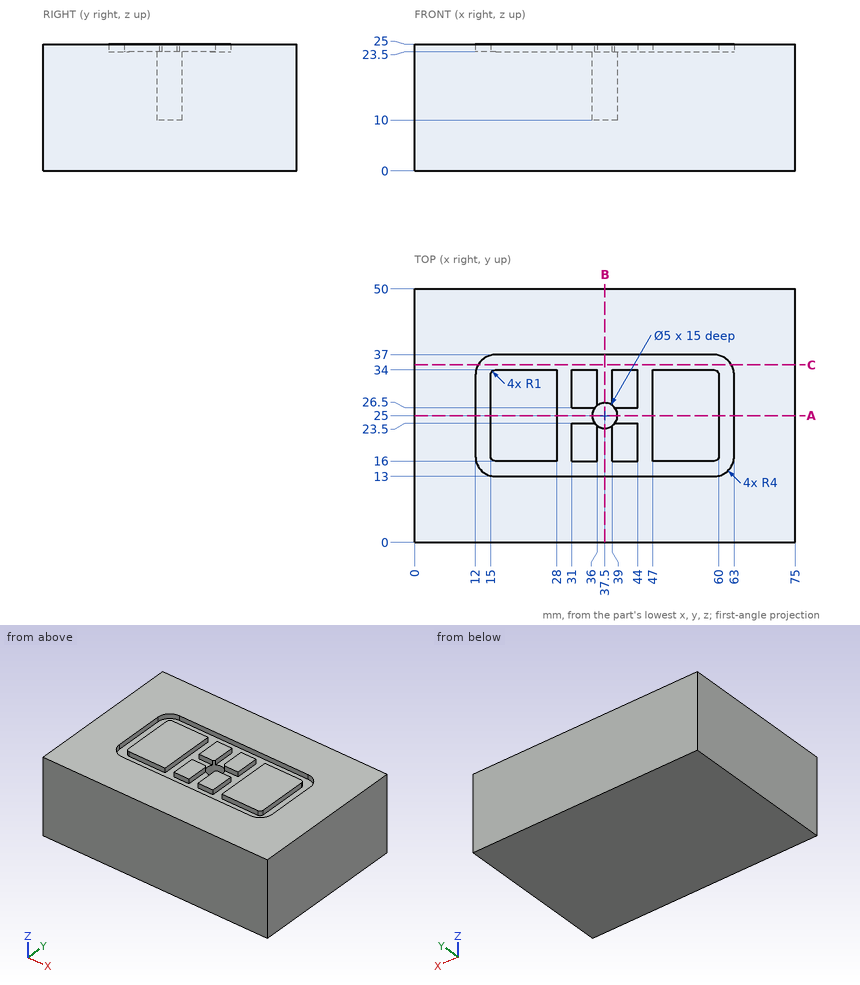
Input: dimensioned drawing with shaded views. Units: mm. Origin: part minimum x, y, z. Coordinates: 2 decimals unless noted, no trailing zeros. Loops run counter-clockwise (first coordinate to the right, second up) from the corner with the lowest first, then second, coordinate; pieces in that order, holes last. Notation, with made-up numbers: M 22,49 L 70,49 A24 ccw 70,82 Z; hole C 87,45.5 d3. An arc over 180 degrees is marked long. One line per item, written item: value.
(1) Section C-C (y = 35). Output: boundary loops of the cut face in (x, z).
Filled in:
outline: M 0,0 L 75,0 L 75,25 L 62.46,25 L 62.46,23.5 L 12.54,23.5 L 12.54,25 L 0,25 Z
(2) Line query: line 1 along Y through (x, z) = (37.5, 13.5); line 2 along X through (y, z) = (25, 20.5); line 3 along Z through (x, y) = (41, 24.5). Output: solid intervals per line, ascending. Write a range as from..to.
Filled in:
line 1: 0..22.5, 27.5..50
line 2: 0..35, 40..75
line 3: 0..23.5
(3) Section B-B (x = 37.5). Output: boundary loops of the cut face in (y, z).
Filled in:
outline: M 0,0 L 50,0 L 50,25 L 37,25 L 37,23.5 L 27.5,23.5 L 27.5,10 L 22.5,10 L 22.5,23.5 L 13,23.5 L 13,25 L 0,25 Z
(4) Pin query (flat end, axial travel): pin 1 (2.5 mm diameter, centred on x = 37.5, y = 26, fed in from +Z). Return the tip coordinate at first contact, or that it passes through.
Filled in:
pin 1: z = 10
(5) Section A-A (y = 25). Output: boundary loops of the cut face in (x, z).
Filled in:
outline: M 0,0 L 75,0 L 75,25 L 63,25 L 63,23.5 L 60,23.5 L 60,25 L 47,25 L 47,23.5 L 40,23.5 L 40,10 L 35,10 L 35,23.5 L 28,23.5 L 28,25 L 15,25 L 15,23.5 L 12,23.5 L 12,25 L 0,25 Z
